from build123d import *

# Parameters (mm, degrees)
SKETCH1_W           = 17.691665124
SKETCH1_H           = 39
SKETCH1_R           = 1.05
BOSS_EXTRUDE1_DEPTH = 6
SKETCH6_R           = 2.5
CUT_EXTRUDE1_DEPTH  = 3.8
FILLET1_R           = 5
FILLET2_R           = 5
SKETCH7_R           = 2.75
CUT_EXTRUDE2_DEPTH  = 0.8


with BuildPart() as part:
    # Sketch1 → Boss-Extrude1 (new body)
    with BuildSketch(Plane(origin=(0, 0, 0), x_dir=(1, 0, 0), z_dir=(0, 1, 0))):
        with Locations((23.537497687, 0)):
            Rectangle(SKETCH1_W, SKETCH1_H)
        with Locations(Location((29.383330249, -12, 0), (0, 0, 270))):
            Circle(SKETCH1_R, mode=Mode.SUBTRACT)
        with BuildLine():
            ThreePointArc((30.383330249, -2), (29.383330249, -3), (28.383330249, -2))
            Line((28.383330249, -2), (28.383330249, 2))
            ThreePointArc((28.383330249, 2), (29.383330249, 3), (30.383330249, 2))
            Line((30.383330249, 2), (30.383330249, -2))
        make_face(mode=Mode.SUBTRACT)
        with Locations(Location((29.383330249, 12, 0), (0, 0, 270))):
            Circle(SKETCH1_R, mode=Mode.SUBTRACT)
    extrude(amount=BOSS_EXTRUDE1_DEPTH)

    # Sketch6 → Cut-Extrude1 (cut)
    with BuildSketch(Plane(origin=(0, 0, 0), x_dir=(-1, 0, 0), z_dir=(0, -1, 0))):
        with Locations((-29.383330249, -12)):
            Circle(SKETCH6_R)
        with Locations((-29.383330249, 12)):
            Circle(SKETCH6_R)
        Polygon((-30.633330249, -9.834936491), (-30.308330249, -10.397853003), (-17.317949192, -2.897853003), (-17.642949192, -2.334936491), align=None)
        Polygon((-30.633330249, 9.834936491), (-30.308330249, 10.397853003), (-17.317949192, 2.897853003), (-17.642949192, 2.334936491), align=None)
    extrude(amount=-CUT_EXTRUDE1_DEPTH, mode=Mode.SUBTRACT)

    # Fillet1
    fillet1_edges = [part.edges().sort_by_distance(p)[0] for p in [
        (32.383330249, 3, 19.5),
        (32.383330249, 3, -19.5),
    ]]
    fillet(fillet1_edges, radius=FILLET1_R)

    # Fillet2
    fillet2_edges = [part.edges().sort_by_distance(p)[0] for p in [
        (14.691665125, 3, 19.5),
        (14.691665125, 3, -19.5),
    ]]
    fillet(fillet2_edges, radius=FILLET2_R)

    # Sketch7 → Cut-Extrude2 (cut)
    with BuildSketch(Plane(origin=(0, 6, 0), x_dir=(1, 0, 0), z_dir=(0, 1, 0))):
        with Locations(Location((29.383330249, 12, 0), (0, 0, 270))):
            Circle(SKETCH7_R)
        with Locations(Location((29.383330249, -12, 0), (0, 0, 90))):
            Circle(SKETCH7_R)
        with BuildLine():
            Line((22.833330249, 16.8), (24.933330249, 16.8))
            ThreePointArc((24.933330249, 16.8), (25.483330249, 16.25), (24.933330249, 15.7))
            Line((24.933330249, 15.7), (22.833330249, 15.7))
            ThreePointArc((22.833330249, 15.7), (22.283330249, 16.25), (22.833330249, 16.8))
        make_face()
        with BuildLine():
            Line((22.833330249, 7.2), (24.933330249, 7.2))
            ThreePointArc((24.933330249, 7.2), (25.483330249, 7.75), (24.933330249, 8.3))
            Line((24.933330249, 8.3), (22.833330249, 8.3))
            ThreePointArc((22.833330249, 8.3), (22.283330249, 7.75), (22.833330249, 7.2))
        make_face()
        with BuildLine():
            Line((22.833330249, -7.2), (24.933330249, -7.2))
            ThreePointArc((24.933330249, -7.2), (25.483330249, -7.75), (24.933330249, -8.3))
            Line((24.933330249, -8.3), (22.833330249, -8.3))
            ThreePointArc((22.833330249, -8.3), (22.283330249, -7.75), (22.833330249, -7.2))
        make_face()
        with BuildLine():
            Line((22.833330249, -16.8), (24.933330249, -16.8))
            ThreePointArc((24.933330249, -16.8), (25.483330249, -16.25), (24.933330249, -15.7))
            Line((24.933330249, -15.7), (22.833330249, -15.7))
            ThreePointArc((22.833330249, -15.7), (22.283330249, -16.25), (22.833330249, -16.8))
        make_face()
    extrude(amount=-CUT_EXTRUDE2_DEPTH, mode=Mode.SUBTRACT)


solid = part.part
Model file for the job. Use its own axes, mm. A direction names the side the tool comes from. Round coordinates to 2 decimals unless told otherwise and drop trailing zeros. Loops run counter-clockwise (first coordinate to the right, second up) from the corner with the lowest first, then second, coordinate; pieces in that order, holes last.
1. Band-saw the part on D-D, the plane y = 4.75. List the corners of the cut face in (x, z).
Check values:
outline: (14.69, -14.5) arc R5 ccw to (19.69, -19.5) - (27.38, -19.5) arc R5 ccw to (32.38, -14.5) - (32.38, 14.5) arc R5 ccw to (27.38, 19.5) - (19.69, 19.5) arc R5 ccw to (14.69, 14.5) - close; hole circle Ø2.1 at (29.38, -12); hole circle Ø2.1 at (29.38, 12); hole (28.38, -2) arc R1 ccw to (30.38, -2) - (30.38, 2) arc R1 ccw to (28.38, 2) - close
2. Mould opens along X. For faces 4 (the cylindrical face through (30.88, 3.042, -18.074)), 5 (the flat face through (24, 5.2, 8)), 6 (the flat face through (23, 3, -19.5)), 7 (the cylindrical face through (31.7, 5.61, -10.52)) say: +X half, -X half, draft (parallel to the pull), parting line (faces both ways), or undercut.
Check values:
face 4: +X half
face 5: undercut
face 6: draft
face 7: undercut
3. Tool access for faces 1 (the flat face through (27.9, 3.8, 10.2)), 2 (the flat face through (29.4, 5.2, -10.8)), 3 (the cylindrical face through (29.4, 3, 3)): list every direction of +Z, -Z, +X, -X, +Y, -Y with a clear straight run to the whole face (end or side of a thin tool).
Check values:
face 1: -Y
face 2: +Y
face 3: +Y, -Y
4. Band-saw the part on C-C, the plane x = 18.25. List the corners of the cut face in (y, z), and give its area (3 significant figures).
Check values:
outline: (0, -19.29) - (6, -19.29) - (6, 19.29) - (0, 19.29) - (0, 3.44) - (3.8, 3.44) - (3.8, 2.69) - (0, 2.69) - (0, -2.69) - (3.8, -2.69) - (3.8, -3.44) - (0, -3.44) - close
area: 226 mm2
5. Band-saw the part on A-A, the plane z = 12. List the corners of the cut face in (x, y).
Check values:
outline: (14.69, 0) - (26.88, 0) - (26.88, 3.8) - (28.33, 3.8) - (28.33, 5.2) - (26.63, 5.2) - (26.63, 6) - (14.69, 6) - close; (30.43, 3.8) - (31.88, 3.8) - (31.88, 0) - (32.38, 0) - (32.38, 6) - (32.13, 6) - (32.13, 5.2) - (30.43, 5.2) - close
6. Band-saw the part on B-B, the plane y = 1.6. List the corners of the cut face in (x, z), and give its area (3 significant figures).
Check values:
outline: (14.69, -14.5) arc R5 ccw to (19.69, -19.5) - (27.38, -19.5) arc R5 ccw to (32.38, -14.5) - (32.38, 14.5) arc R5 ccw to (27.38, 19.5) - (19.69, 19.5) arc R5 ccw to (14.69, 14.5) - close; hole (17.32, -2.9) - (28.85, -9.56) arc R2.5 ccw (long way) to (30.63, -9.83) - (17.64, -2.33) - close; hole (17.32, 2.9) - (17.64, 2.33) - (30.63, 9.83) arc R2.5 ccw (long way) to (28.85, 9.56) - close; hole (28.38, -2) arc R1 ccw to (30.38, -2) - (30.38, 2) arc R1 ccw to (28.38, 2) - close
area: 600 mm2
7. Wall check: probe 1 along X at (y, z) = (4.4, -12); probe 2 along Z at (x, y) = (24.25, 2.35); probe 3 along Z at (x, y) = (19.5, 2.4). Give the ranges that are in metal, low to high.
Check values:
probe 1: x = 14.69 to 28.33, 30.43 to 32.38
probe 2: z = -19.5 to -6.9, -6.15 to 6.15, 6.9 to 19.5
probe 3: z = -19.5 to -4.16, -3.41 to 3.41, 4.16 to 19.5
8. Drop flat-ended pins along their axis: P1, Ø2.5, axis at x = 29.38, z = 12, coming from the -Y side; P2, Ø3, axis at x = 29, z = -12, coming from the +Y side. Give the stop position or say it passes through.
Check values:
P1: stops at y = 3.8
P2: stops at y = 5.2
